```python
from build123d import *

# Parameters (mm, degrees)
SKETCH1_R           = 1
BOSS_EXTRUDE1_DEPTH = 1.5


with BuildPart() as part:
    # Sketch1 → Boss-Extrude1 (new body)
    # profile 1 of 3: a face of its own
    with BuildSketch(Plane(origin=(0, 0, 0), x_dir=(1, 0, 0), z_dir=(0, 1, 0))):
        with BuildLine():
            ThreePointArc((-38.479582276, 15.672906391), (-38.624558781, 14.925318383), (-39.038470107, 14.28611307))
            Line((-39.038470107, 14.28611307), (-16.611056788, 14.505213721))
            Line((-16.611056788, 14.505213721), (-16.611056788, 15.164223273))
            Line((-16.611056788, 15.164223273), (-40.063758895, 17.629201593))
            ThreePointArc((-40.063758895, 17.629201593), (-38.925290354, 16.931547173), (-38.479582276, 15.672906391))
        make_face()
    # profile 2 of 3: a face of its own
    with BuildSketch(Plane(origin=(0, 0, 0), x_dir=(1, 0, 0), z_dir=(0, 1, 0))):
        with BuildLine():
            ThreePointArc((-40.479582276, 17.672906391), (-41.704327148, 17.254045221), (-42.41607395, 16.172906391))
            ThreePointArc((-42.41607395, 16.172906391), (-42.479582276, 15.672906391), (-42.41607395, 15.172906391))
            ThreePointArc((-42.41607395, 15.172906391), (-40.987470858, 13.738468698), (-39.038470107, 14.28611307))
            ThreePointArc((-39.038470107, 14.28611307), (-38.624558781, 14.925318383), (-38.479582276, 15.672906391))
            ThreePointArc((-38.479582276, 15.672906391), (-38.925290354, 16.931547173), (-40.063758895, 17.629201593))
            Line((-40.063758895, 17.629201593), (-40.479582276, 17.672906391))
        make_face()
        with Locations(Location((-40.479582276, 15.672906391, 0), (0, 0, 270))):
            Circle(SKETCH1_R, mode=Mode.SUBTRACT)
    # profile 3 of 3: a face of its own
    with BuildSketch(Plane(origin=(0, 0, 0), x_dir=(1, 0, 0), z_dir=(0, 1, 0))):
        with BuildLine():
            Line((-42.41607395, 16.172906391), (-44.35607395, 16.172906391))
            Line((-44.35607395, 16.172906391), (-44.35607395, 15.172906391))
            Line((-44.35607395, 15.172906391), (-42.41607395, 15.172906391))
            ThreePointArc((-42.41607395, 15.172906391), (-42.479582276, 15.672906391), (-42.41607395, 16.172906391))
        make_face()
    extrude(amount=BOSS_EXTRUDE1_DEPTH)


solid = part.part
```
Here's how the part is built. I have some questions about the finished solid (model axes, mm). A direction names the side the tool comes from. Coordinates: 2 decimals unless noted, no trailing zeros. Order: outer loops, then holes, each group sorted by start corner. A loop starts at its lowest first (then second) coordinate and runs counter-clockwise, first axis right, second up.
1) I need wall thicknesses on line 1 (X direction, y = 0.8, z = -15); line 2 (Z direction, x = -20.75, y = 0.75); line 3 (Z direction, x = -41, y = 0.25). Which ranges of each line are inside material? Lowest first, please.
2) Imagine slicing it at B-B on y = 0.95. List the corners of the cut face in (x, z) for me, and give its area (3 significant figures).
3) Imagine slicing it at C-C on x = -24.5. List the corners of the cut face in (y, z) for me.
4) Imagine slicing it at A-A on z = -15.4. List the corners of the cut face in (x, y) for me, and give its area (3 significant figures).
5) Which directions (+Z, -Z, +X, -X, +Y, -Y) give clear straight access to the entire face, cutting with the end or side of a thin tool? Please do faces 1 (the face through (-43, 1, -16.173)), 2 (the face through (-41.456, 0.74, -15.89)), 3 (the face through (-43, 1, -15.173)).
6) Imagine slicing it at D-D on x = -38.75. List the corners of the cut face in (y, z) for me.
Response values:
1. line 1: x = -42.36 to -41.22, -39.74 to -16.61
1. line 2: z = -15.6 to -14.46
1. line 3: z = -17.6 to -16.53, -14.82 to -13.74
2. outline: (-44.36, -16.17) - (-42.42, -16.17) arc R2 ccw to (-40.48, -17.67) - (-16.61, -15.16) - (-16.61, -14.51) - (-39.04, -14.29) arc R2 ccw to (-42.42, -15.17) - (-44.36, -15.17) - close; hole circle Ø2 at (-40.48, -15.67)
2. area: 54.1 mm2
3. outline: (0, -15.99) - (1.5, -15.99) - (1.5, -14.43) - (0, -14.43) - close
4. outline: (-44.36, 0) - (-41.44, 0) - (-41.44, 1.5) - (-44.36, 1.5) - close; (-39.52, 0) - (-18.85, 0) - (-18.85, 1.5) - (-39.52, 1.5) - close
4. area: 35.4 mm2
5. face 1: -Z, -X, +Y, -Y
5. face 2: +Y, -Y
5. face 3: +Z, -X, +Y, -Y
6. outline: (0, -17.49) - (1.5, -17.49) - (1.5, -14.29) - (0, -14.29) - close
